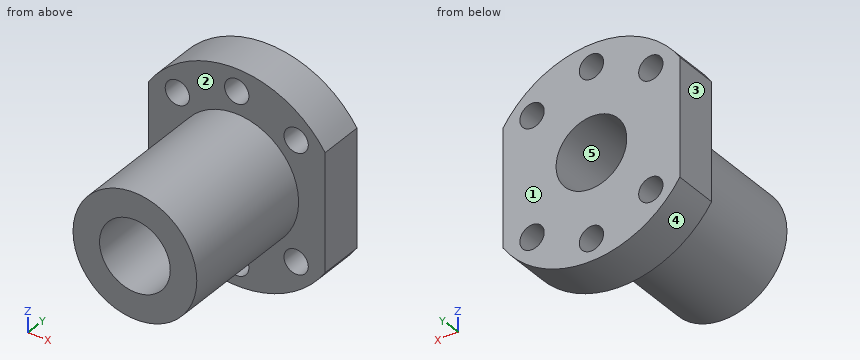
```python
from build123d import *

# Parameters (mm, degrees)
F1_DEPTH = 10
F2_R     = 14
F3_DEPTH = 32
F4_R     = 8
F5_DEPTH = 42.001
F6_R     = 2.75
F7_DEPTH = 42.001


with BuildPart() as f1:
    # F0 (on Front) → F1 (new body)
    with BuildSketch(Plane.XZ):
        with BuildLine():
            Line((-20, 13.266499), (-20, -13.266499))
            ThreePointArc((-20, -13.266499), (0, -24), (20, -13.266499))
            Line((20, -13.266499), (20, 13.266499))
            ThreePointArc((20, 13.266499), (0, 24), (-20, 13.266499))
        make_face()
    extrude(amount=F1_DEPTH)

    # F2 (on face) → F3 (join)
    with BuildSketch(Plane.XZ.offset(10)):
        Circle(F2_R)
    extrude(amount=F3_DEPTH)

    # F4 (on face) → F5 (cut, through all)
    with BuildSketch(Plane.XZ.offset(42)):
        Circle(F4_R)
    extrude(amount=-F5_DEPTH, mode=Mode.SUBTRACT)

    # F6 (on face) → F7 (cut, through all)
    with BuildSketch(Plane(origin=(0, 0, 0), x_dir=(-1, 0, 0), z_dir=(0, 1, 0))):
        with Locations((0, 19)):
            Circle(F6_R)
        with Locations((-13.435029, 13.435029)):
            Circle(F6_R)
        with Locations((-13.435029, -13.435029)):
            Circle(F6_R)
        with Locations((0, -19)):
            Circle(F6_R)
        with Locations((13.435029, -13.435029)):
            Circle(F6_R)
        with Locations((13.435029, 13.435029)):
            Circle(F6_R)
    extrude(amount=-F7_DEPTH, mode=Mode.SUBTRACT)


solid = f1.part
```
Geometry check sheet. Reference: the model listing, model coordinates, mm. Face numbers are marked on the shaded views. A direction names the side the tool comes from. Round coordinates to 2 decimals unless told otherwise and drop trailing zeros. Order: outer loops, then holes, each group sorted by start corner. A loop starts at its lowest first (then second) coordinate and runs counter-clockwise, first axis right, second up. Notation, with made-up numbers: (56, 4) - (77, 4) arc R24 ccw to (77, 39) - close; hole circle Ø2 at (39.25, 43). An arc over 180 degrees is marked (long way). Use a Markdown table: item, result. Add a question column.
1) Section check D-D (y = -33). Record the cut outline in (x, z), then the cut area to 3 significant figures.
2) Mould release check, pull along X, two halves, no side actions. Record for the marked faces 3, 4 and 5: released by +X, released by -X, zero draft, split by the parting line, or undercut.
3) Section check B-B (z = 0). Record the cut outline in (x, y).
4) Set-up check for the marked faces 1 and 2: record each of +Z, -Z, +X, -X, +Y, -Y from which the full face is reachable in a straight line by a thin tool's end or side.
5) Section check C-C (x = 5.5). Record the cut outline in (y, z).
6) Thickness scan on line 1 along Y through (x, z) = (-18, -3.5); line 2 along Z through (x, y) = (3, -24); line 3 along X through (y, z) = (-7.5, -18.5). Record the ranges inside material, lowest first.
7) Section check A-A (x = 0). Record the cut outline in (y, z), then the cut area to 3 significant figures.
8) Gauge pin test, flat ends, axial feed: P1, Ø10, axis at y = -31, z = 12.5, coming from the +X side; P2, Ø4.5, axis at x = 0, z = -19, coming from the +Y side; P3, Ø4, axis at x = 3.5, y = -9, coming from the +Z side; P4, Ø10, axis at x = -7, y = -9.5, coming from the -Z side. Record the tip position at first contact, or that the pin passes through.
Established:
| question | item | result |
|---|---|---|
| 1 | outline | circle Ø28 at (0, 0); hole circle Ø16 at (0, 0) |
| 1 | area | 415 mm2 |
| 2 | face 3 | released by -X |
| 2 | face 4 | split by the parting line |
| 2 | face 5 | undercut |
| 3 | outline | (-20, -10) - (-14, -10) - (-14, -42) - (-8, -42) - (-8, 0) - (-20, 0) - close; (8, -42) - (14, -42) - (14, -10) - (20, -10) - (20, 0) - (8, 0) - close |
| 4 | face 1 | +Z, -Z, +X, -X, +Y |
| 4 | face 2 | -Y |
| 5 | outline | (-42, -12.87) - (-10, -12.87) - (-10, -23.36) - (0, -23.36) - (0, -5.81) - (-42, -5.81) - close; (-42, 5.81) - (0, 5.81) - (0, 23.36) - (-10, 23.36) - (-10, 12.87) - (-42, 12.87) - close |
| 6 | line 1 | -10 to 0 |
| 6 | line 2 | -13.67 to -7.42, 7.42 to 13.67 |
| 6 | line 3 | -15.29 to -2.7, 2.7 to 15.29 |
| 7 | outline | (-42, -14) - (-10, -14) - (-10, -16.25) - (0, -16.25) - (0, -8) - (-42, -8) - close; (-42, 8) - (0, 8) - (0, 16.25) - (-10, 16.25) - (-10, 14) - (-42, 14) - close; (-10, -24) - (0, -24) - (0, -21.75) - (-10, -21.75) - close; (-10, 21.75) - (0, 21.75) - (0, 24) - (-10, 24) - close |
| 7 | area | 594 mm2 |
| 8 | P1 | x = 11.82 |
| 8 | P2 | through |
| 8 | P3 | z = 23.95 |
| 8 | P4 | z = -23.92 |
